from build123d import *

# Parameters (mm, degrees)
SKETCH1_R           = 5
SKETCH1_R_2         = 1
BOSS_EXTRUDE1_DEPTH = 3.5
BOSS_EXTRUDE2_DEPTH = 7.9
SKETCH3_W           = 20
SKETCH3_H           = 25.3
SKETCH3_R           = 5
BOSS_EXTRUDE3_DEPTH = 2
FILLET1_R           = 2
FILLET2_R           = 1


with BuildPart() as part:
    # Sketch1 → Boss-Extrude1 (new body)
    with BuildSketch(Plane(origin=(0, 0, 0), x_dir=(0, 0, -1), z_dir=(1, 0, 0))):
        with BuildLine():
            Line((10, -20.2), (10, 20.2))
            ThreePointArc((10, 20.2), (0, 30.2), (-10, 20.2))
            Line((-10, 20.2), (-10, -20.2))
            ThreePointArc((-10, -20.2), (0, -30.2), (10, -20.2))
        make_face()
        Circle(SKETCH1_R, mode=Mode.SUBTRACT)
        with Locations((0, 20.2)):
            Circle(SKETCH1_R_2, mode=Mode.SUBTRACT)
        with Locations((0, -20.2)):
            Circle(SKETCH1_R_2, mode=Mode.SUBTRACT)
    extrude(amount=BOSS_EXTRUDE1_DEPTH)

    # Sketch2 → Boss-Extrude2 (add)
    with BuildSketch(Plane(origin=(3.5, 0, 0), x_dir=(0, 0, -1), z_dir=(1, 0, 0))):
        Polygon((-9.988159657, 0), (-4.994079828, 8.65), (10, 8.65), (10, 12.65), (-10, 12.65), (-10, -12.65), (10, -12.65), (10, -8.65), (-4.994079828, -8.65), align=None)
    extrude(amount=BOSS_EXTRUDE2_DEPTH)

    # Sketch3 → Boss-Extrude3 (add)
    with BuildSketch(Plane(origin=(11.4, 0, 0), x_dir=(0, 0, -1), z_dir=(1, 0, 0))):
        Rectangle(SKETCH3_W, SKETCH3_H)
        Circle(SKETCH3_R, mode=Mode.SUBTRACT)
    extrude(amount=BOSS_EXTRUDE3_DEPTH)

    # Fillet1
    fillet1_edges = [part.edges().sort_by_distance(p)[0] for p in [
        (7.45, 0, 9.988159657),
        (3.5, -12.65, 0),
        (3.5, 12.65, 0),
    ]]
    fillet(fillet1_edges, radius=FILLET1_R)

    # Fillet2
    fillet2_edges = [part.edges().sort_by_distance(p)[0] for p in [
        (3.5, 0, -10),
        (11.4, -8.65, -2.502960086),
        (7.45, -8.65, -10),
        (11.4, 4.825, 7.202444608),
        (3.5, 8.65, -2.502960086),
        (7.45, 8.65, -10),
        (11.4, 8.65, -2.502960086),
        (3.5, -8.65, -2.502960086),
        (3.5, 4.825, 7.202444608),
        (11.4, 0, 5),
        (11.4, 0, -10),
        (3.5, -4.825, 7.202444608),
        (3.5, 0, 9.67875858),
        (11.4, -4.825, 7.202444608),
        (11.4, 0, 9.67875858),
        (3.5, 0, 5),
    ]]
    fillet(fillet2_edges, radius=FILLET2_R)


solid = part.part
Can you work these out from the model? Positions are in its coordinate system, mm. A direction names the side the tool comes from. Coordinates: 2 decimals unless noted, no trailing zeros. Order: outer loops, then holes, each group sorted by start corner. A loop starts at its lowest first (then second) coordinate and runs counter-clockwise, first axis right, second up. Notation, with made-up numbers: (66.5, 19.25) -> (122.5, 19.25) arc R23 ccw to (122.5, 43.25) -> close; hole circle Ø8 at (63, 1.25). An arc over 180 degrees is marked (long way). Use one line per item in the form item = value.
Q1. Imagine slicing it at A-A, the plane x = 1. List the corners of the cut face in (y, z) for me, then the cut area to 3 significant figures.
From the geometry:
outline = (-20.2, -10) -> (20.2, -10) arc R10 ccw to (20.2, 10) -> (-20.2, 10) arc R10 ccw to start; hole circle Ø2 at (-20.2, 0); hole circle Ø10 at (0, 0); hole circle Ø2 at (20.2, 0)
area = 1,040 mm²
Q2. Imagine slicing it at C-C, the plane z = -7. List the corners of the cut face in (x, y) for me.
From the geometry:
outline = (0, -27.34) -> (3.5, -27.34) -> (3.5, -14.65) arc R2 cw to (5.5, -12.65) -> (13.4, -12.65) -> (13.4, 12.65) -> (5.5, 12.65) arc R2 cw to (3.5, 14.65) -> (3.5, 27.34) -> (0, 27.34) -> close; hole (3.5, -7.65) arc R1 ccw to (4.5, -8.65) -> (10.4, -8.65) arc R1 ccw to (11.4, -7.65) -> (11.4, 7.65) arc R1 ccw to (10.4, 8.65) -> (4.5, 8.65) arc R1 ccw to (3.5, 7.65) -> close
Q3. Will these pins go through, and if not, where does the flat tip stop? P1, Ø4, axis at x = 7.5, z = -0.5, coming from the -Y side; P2, Ø8, axis at y = 23.5, z = 2.5, coming from the +X side; P3, Ø8, axis at y = 0, z = 0, coming from the -X side; P4, Ø4.5, axis at x = 8, z = 0, coming from the +Y side.
From the geometry:
P1 = -12.65
P2 = 3.5
P3 = through
P4 = 12.65
Q4. I need wall thicknesses on L1, parallel to Y at x = 7.75, z = 4; L2, parallel to Y at x = 1.2, z = 0; L3, parallel to X at y = 15.5, z = -7. Which ranges of each line are inside material? Lowest first, please.
From the geometry:
L1 = -12.65 to -8.65, 8.65 to 12.65
L2 = -30.2 to -21.2, -19.2 to -5, 5 to 19.2, 21.2 to 30.2
L3 = 0 to 3.5
Q5. We'd pull the mould along X, two halves only. Please class faces 4 (the face through (13.4, 3, -4.3)), 5 (the face through (3.199, 0.107, -9.715)), 6 (the face through (1.7, 30.2, -0.2)): released by +X, released by -X, zero draft, split by the parting line, or undercut.
From the geometry:
face_4 = released by +X
face_5 = undercut
face_6 = zero draft
Q6. Imagine slicing it at D-D, the plane z = 0. Give the number of separate pieces and of enclosed holes in the cut face, then the cut area to 3 significant figures.
From the geometry:
separate_pieces = 4
enclosed_holes = 0
area = 258 mm²
Q7. Imagine slicing it at B-B, the plane x = 9.5. List the corners of the cut face in (y, z) for me, then the cut area to 3 significant figures.
From the geometry:
outline = (-12.65, -10) -> (-9.65, -10) arc R1 ccw to (-8.65, -9) -> (-8.65, 4.99) -> (-1, 9.41) arc R2 cw to (1, 9.41) -> (8.65, 4.99) -> (8.65, -9) arc R1 ccw to (9.65, -10) -> (12.65, -10) -> (12.65, 10) -> (-12.65, 10) -> close
area = 203 mm²
Q8. Which directions (+Z, -Z, +X, -X, +Y, -Y) give clear straight access to the entire face, cutting with the end or side of a thin tool? Please do faces 1 (the face through (1.7, -30.2, 0.2)), 2 (the face through (7, 8.65, -2)), 3 (the face through (9, 12.65, 0)).
From the geometry:
face_1 = +X, -X, -Y
face_2 = -Z
face_3 = +Z, -Z, +X, +Y
